Answer from the drawing. Dimensions are ordinates in mm from the lowest x, y and z of the part. Round coordinates to 2 decimals unless told otherwise and drop trailing zeros. Write each loop counter-clockwise with the first axis right and the second up, starting at its lowest first coordinate (ties: lowest second). Pieces come first, ordered by that corner, then holes.
1. Find section A-A (x = 69). Write down the section's boundary in (y, z) (1 decimal).
2. Find section D-D (x = 23). Write down the section's boundary in (y, z) (1 decimal).
3. Flat-ended cylindrical pins translate along their axes: pin 1 Ø1 at (y, z) = (1.5, 52.5) entering from -X; pin 2 Ø1 at (x, y) = (4, 2) entering from +Z (1 decimal); pin 3 Ø1 at (x, y) = (5.5, 2.5) entering from -Z. Find the tip coordinate at first contact, or state that the pin passes through.
4. Find section C-C (z = 78.5). Write down the section's boundary in (x, y) (1 decimal).
5. Straight lines are drawn through the part: probe 1 along X at (y, z) = (3.05, 51.5); probe 2 along Z at (x, y) = (50, 0.8); probe 3 along Z at (x, y) = (66, 1.15) (1 decimal). For each, find the intervals that lie inside material, in ascending order.
6. Find section B-B (y = 2.1). Write down the section's boundary in (x, z) (1 decimal).
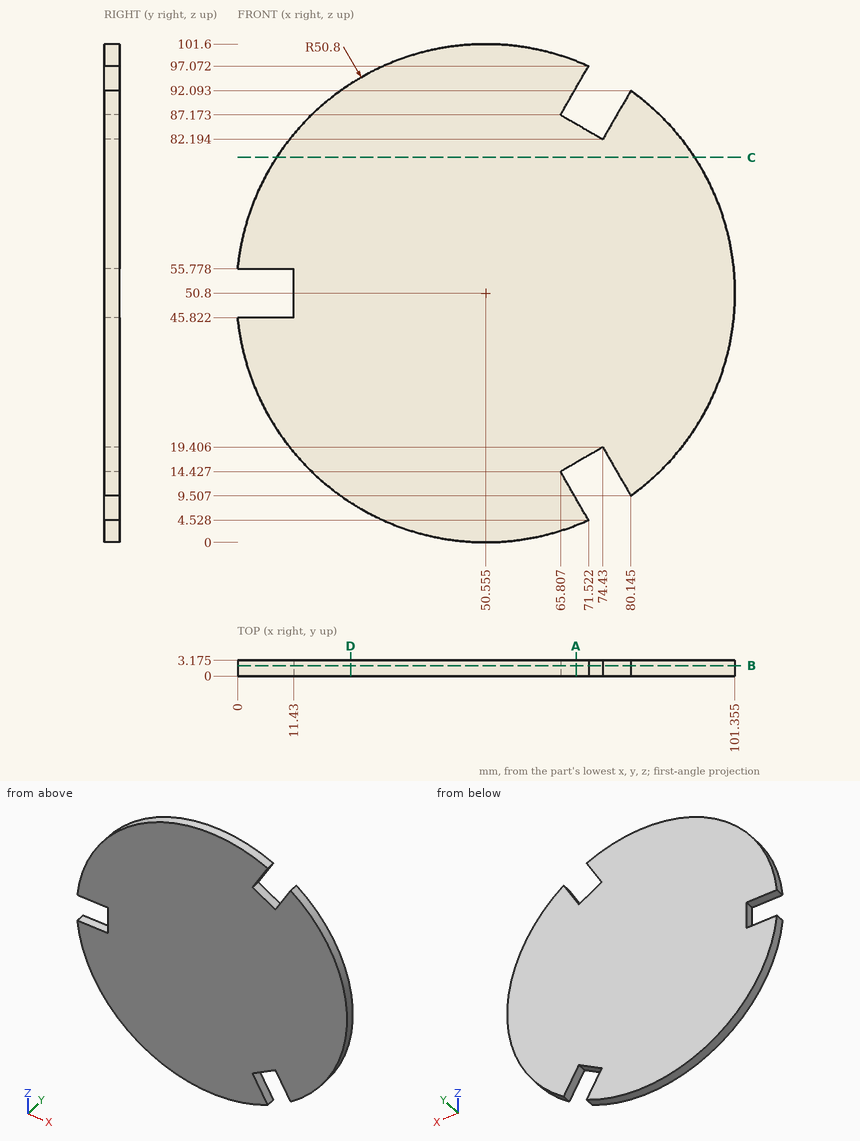
Worked answers:
1. outline: (0, 3.5) - (3.2, 3.5) - (3.2, 8.9) - (0, 8.9) - close; (0, 16.3) - (3.2, 16.3) - (3.2, 85.3) - (0, 85.3) - close; (0, 92.7) - (3.2, 92.7) - (3.2, 98.1) - (0, 98.1) - close
2. outline: (0, 8.1) - (3.2, 8.1) - (3.2, 93.5) - (0, 93.5) - close
3. pin 1: stops at x = 11.43
3. pin 2: stops at z = 72.2
3. pin 3: stops at z = 26.4
4. outline: (8, 0) - (93.1, 0) - (93.1, 3.2) - (8, 3.2) - close
5. probe 1: x = 11.43 to 101.35
5. probe 2: z = 0 to 101.6
5. probe 3: z = 2.4 to 14.1, 14.5 to 87.1, 87.5 to 99.2
6. outline: (0, 45.8) arc R50.8 ccw to (71.5, 4.5) - (65.8, 14.4) - (74.4, 19.4) - (80.1, 9.5) arc R50.8 ccw to (80.1, 92.1) - (74.4, 82.2) - (65.8, 87.2) - (71.5, 97.1) arc R50.8 ccw to (0, 55.8) - (11.4, 55.8) - (11.4, 45.8) - close
